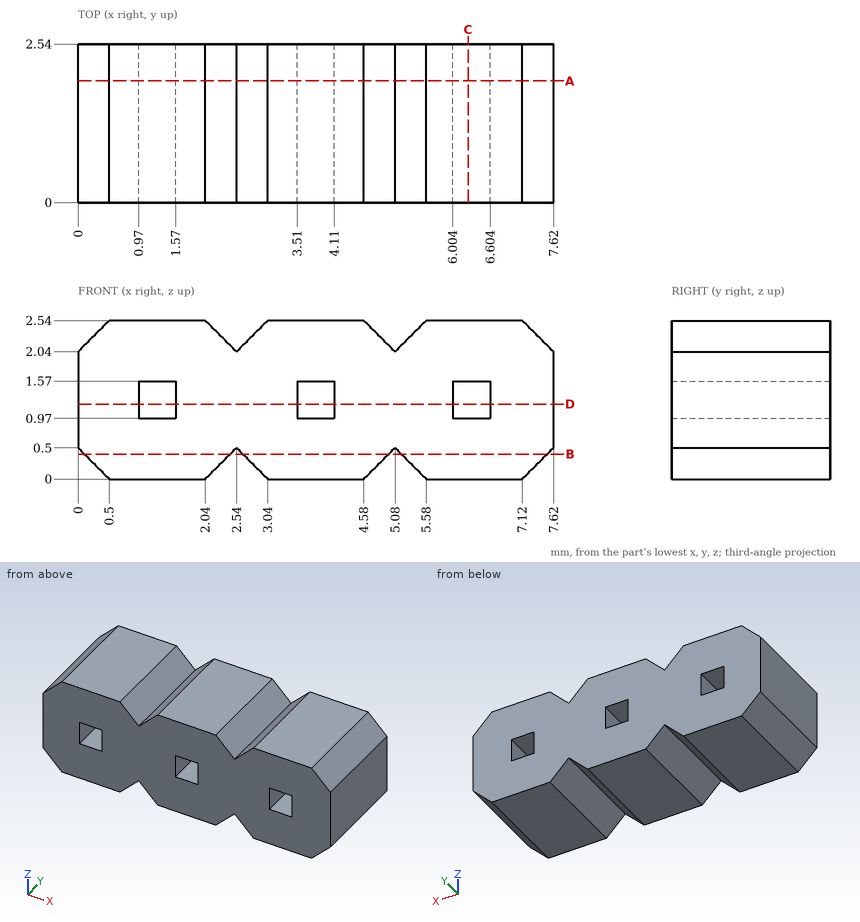
Job drawing, mm, ordinate dimensions from the low corner. One solid piece. Coordinates: 2 decimals unless noted, no trailing zeros. Write each loop counter-clockwise with the first axis right and the second up, starting at its lowest first coordinate (ties: lowest second). Pieces come first, ordered by that corner, then holes.
Item 1: Slice it at B-B (z = 0.4). Write the cut outline in (x, y).
Item 2: Slice it at A-A (y = 1.95). Count the separate pieces of the cut face and the enclosed holes in it, and give its area (3 significant figures).
Item 3: Probe line 1 (X direction, y = 1.6, z = 1.5); line 2 (Z direction, x = 3.75, y = 2); line 3 (X direction, y = 2, z = 0.25). List the from-to ranges inside material, lowest first.
Item 4: Slice it at D-D (z = 1.2). Write the cut outline in (x, y).
Item 5: Slice it at C-C (x = 6.25). Write the cut outline in (y, z).
Results found:
1. outline: (0.1, 0) - (2.44, 0) - (2.44, 2.54) - (0.1, 2.54) - close; (2.64, 0) - (4.98, 0) - (4.98, 2.54) - (2.64, 2.54) - close; (5.18, 0) - (7.52, 0) - (7.52, 2.54) - (5.18, 2.54) - close
2. separate pieces: 1
2. enclosed holes: 3
2. area: 16.8 mm2
3. line 1: x = 0 to 0.97, 1.57 to 3.51, 4.11 to 6, 6.6 to 7.62
3. line 2: z = 0 to 0.97, 1.57 to 2.54
3. line 3: x = 0.25 to 2.29, 2.79 to 4.83, 5.33 to 7.37
4. outline: (0, 0) - (0.97, 0) - (0.97, 2.54) - (0, 2.54) - close; (1.57, 0) - (3.51, 0) - (3.51, 2.54) - (1.57, 2.54) - close; (4.11, 0) - (6, 0) - (6, 2.54) - (4.11, 2.54) - close; (6.6, 0) - (7.62, 0) - (7.62, 2.54) - (6.6, 2.54) - close
5. outline: (0, 0) - (2.54, 0) - (2.54, 0.97) - (0, 0.97) - close; (0, 1.57) - (2.54, 1.57) - (2.54, 2.54) - (0, 2.54) - close
